For this review, take the finished solid that the model builds, in its own axes (mm). Face numbers are marked on the shaded views. A direction names the side the tool comes from. Round coordinates to 2 decimals unless told otherwise and drop trailing zeros. Loops run counter-clockwise (first coordinate to the right, second up) from the corner with the lowest first, then second, coordinate; pieces in that order, holes last.
```python
from build123d import *

# Parameters (mm, degrees)
SZKIC1_R                         = 6.5
DODANIE_WYCI_GNI_CIE1_DEPTH      = 30
ZAOKR_GLENIE1_R                  = 2
SZKIC2_R                         = 4.5
WYTNIJ_WYCI_GNI_CIE1_DEPTH       = 30
SZKIC3_R                         = 16
DODANIE_WYCI_GNI_CIE2_DEPTH      = 14
ZAOKR_GLENIE2_R                  = 7
SZKIC4_R                         = 18
DODANIE_WYCI_GNI_CIE3_DEPTH      = 4
DODANIE_WYCI_GNI_CIE4_REACH      = 61.397
DODANIE_WYCI_GNI_CIE4_END_RADIUS = 18
SZKIC5_W                         = 36
SZKIC5_H                         = 4
WYTNIJ_WYCI_GNI_CIE2_REACH       = 57.642


with BuildPart() as part:
    # Szkic1 → Dodanie-wyciągnięcie1 (new body)
    with BuildSketch(Plane.XY):
        Circle(SZKIC1_R)
    extrude(amount=DODANIE_WYCI_GNI_CIE1_DEPTH)

    # Zaokrąglenie1
    zaokr_glenie1_edges = [part.edges().sort_by_distance(p)[0] for p in [
        (-6.5, 0, 30),
    ]]
    fillet(zaokr_glenie1_edges, radius=ZAOKR_GLENIE1_R)

    # Szkic2 → Wytnij-wyciągnięcie1 (cut)
    with BuildSketch(Plane(origin=(0, 0, 0), x_dir=(-1, 0, 0), z_dir=(0, 0, -1))):
        Circle(SZKIC2_R)
    extrude(amount=-WYTNIJ_WYCI_GNI_CIE1_DEPTH, mode=Mode.SUBTRACT)

    # Szkic3 → Dodanie-wyciągnięcie2 (add)
    with BuildSketch(Plane(origin=(0, 0, 0), x_dir=(-1, 0, 0), z_dir=(0, 0, -1))):
        Circle(SZKIC3_R)
    extrude(amount=DODANIE_WYCI_GNI_CIE2_DEPTH)

    # Zaokrąglenie2
    zaokr_glenie2_edges = [part.edges().sort_by_distance(p)[0] for p in [
        (16, 0, 0),
    ]]
    fillet(zaokr_glenie2_edges, radius=ZAOKR_GLENIE2_R)

    # Szkic4 → Dodanie-wyciągnięcie3 (add)
    with BuildSketch(Plane(origin=(0, 0, -14), x_dir=(-1, 0, 0), z_dir=(0, 0, -1))):
        Circle(SZKIC4_R)
    extrude(amount=DODANIE_WYCI_GNI_CIE3_DEPTH)

    # Dodanie-wyciągnięcie4: up to this cylinder (the profile starts outside it)
    dodanie_wyci_gni_cie4_end = Plane(origin=(0, 0, -16), z_dir=(0, 0, 1)) * Cylinder(DODANIE_WYCI_GNI_CIE4_END_RADIUS, 159.794, mode=Mode.PRIVATE)
    # Szkic5 → Dodanie-wyciągnięcie4 (add, up to the surface)
    with BuildSketch(Plane(origin=(0, 30, 0), x_dir=(1, 0, 0), z_dir=(0, 1, 0)), mode=Mode.PRIVATE) as dodanie_wyci_gni_cie4_sk1:
        with Locations((0, 16)):
            Rectangle(SZKIC5_W, SZKIC5_H)
    dodanie_wyci_gni_cie4_tool1 = extrude(dodanie_wyci_gni_cie4_sk1.sketch, amount=-DODANIE_WYCI_GNI_CIE4_REACH, mode=Mode.PRIVATE) - dodanie_wyci_gni_cie4_end
    add(dodanie_wyci_gni_cie4_tool1.solids().sort_by_distance((0, 30, -16))[0])

    # Szkic6 → Wytnij-wyciągnięcie2 (cut, up to next)
    with BuildSketch(Plane(origin=(18, 0, 0), x_dir=(0, 0, -1), z_dir=(1, 0, 0)), mode=Mode.PRIVATE) as wytnij_wyci_gni_cie2_sk1:
        Polygon((18, 30), (14, 24), (14, 30), align=None)
    wytnij_wyci_gni_cie2_tool1 = extrude(wytnij_wyci_gni_cie2_sk1.sketch, amount=-WYTNIJ_WYCI_GNI_CIE2_REACH, mode=Mode.PRIVATE) & part.part
    add(wytnij_wyci_gni_cie2_tool1.solids().sort_by_distance((18, 28, -15.333333))[0], mode=Mode.SUBTRACT)


solid = part.part
```
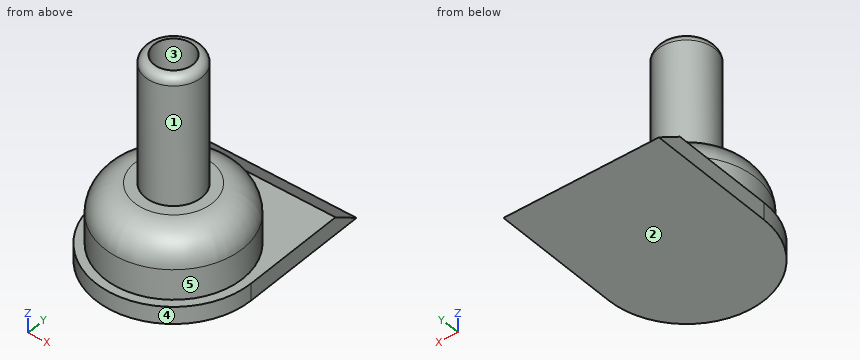
(1) Add section A-A (x = 0). Give the boundary of the cut face in (y, z).
(2) For L1, parallel to Y at x = 0, z = 13; L2, parallel to Z at x = 1, y = 8.5; L3, parallel to Z at x = 8, y = 14, list the stretches that pass through material, from the lowest coordinate up.
(3) Insertion check: pin 1 Ø2 at (y, z) = (12, -6.5) entering from -X; pin 2 Ø12 at (y, z) = (-8, 10.5) entering from +X; pin 3 Ø3 at (y, z) = (5, 17.5) entering from -X; pin 4 Ø14.5 at (x, y) = (3, 0) entering from +Z. Each pin has a flat end and moves straight along its axis. Give the tip position at first contact, or say it passes through.
(4) Add section C-C (z = -15). Give the boundary of the cut face in (x, y).
(5) For the marked faces 4 and 5, list the 3-axis set-ups (+Z, -Z, +X, -X, +Y, -Y) from which the entire face can be reached by the end or side of a thin tool; tool diameter is ignored.
(6) Add section B-B (z = 23). Give the boundary of the cut face in (x, y), plus the area to 3 significant figures.
(7) The part is to be moulded in two halves that separate along Y. For the marked faces 1, 2 and 3, say which applies: pulls with the +Y half, pulls with the -Y half, needs draft (parallel to the pull), parting line crosses it, or undercut.
(8) Add section D-D (z = -5.5). Give the boundary of the cut face in (x, y).
Outcome:
1. outline: (-18, -18) - (30, -18) - (24, -14) - (16, -14) - (16, -7) arc R7 ccw to (9, 0) - (6.5, 0) - (6.5, 28) arc R2 ccw to (4.5, 30) - (4.5, 0) - (-4.5, 0) - (-4.5, 30) arc R2 ccw to (-6.5, 28) - (-6.5, 0) - (-9, 0) arc R7 ccw to (-16, -7) - (-16, -14) - (-18, -14) - close
2. L1: y = -6.5 to -4.5, 4.5 to 6.5
2. L2: z = -18 to 0
2. L3: z = -18 to -14
3. pin 1: stops at x = -11.6
3. pin 2: stops at x = 6.18
3. pin 3: stops at x = -5.48
3. pin 4: stops at z = 30
4. outline: (-18, 0) arc R18 ccw to (18, 0) - (18, 25.5) - (-18, 25.5) - close
5. face 4: +Z, -Z, -Y
5. face 5: +Z
6. outline: circle Ø13 at (0, 0); hole circle Ø9 at (0, 0)
6. area: 69.1 mm2
7. face 1: parting line crosses it
7. face 2: needs draft
7. face 3: undercut
8. outline: circle Ø31.67 at (0, 0)
